Read the model definition and answer for the solid it produces. Units are mm, in the model's axes. A direction names the side the tool comes from. Coordinates: 2 decimals unless noted, no trailing zeros. Write each loop counter-clockwise with the first axis right and the second up, starting at its lowest first coordinate (ties: lowest second). Pieces come first, ordered by that corner, then holes. Notation, with made-up numbers: (33, 24) - (44, 24) arc R20 ccw to (44, 59) - close; hole circle Ø6 at (-28.75, 8). An arc over 180 degrees is marked (long way). Return JSON: item names as keys, results as strings.
Autodesk Inventor part; units mm, degrees
ref_plane "YZ Plane" through (0, 0, 0) normal (1, 0, 0) x (0, 1, 0)
ref_plane "XZ Plane" through (0, 0, 0) normal (0, 1, 0) x (-1, 0, 0)
ref_plane "XY Plane" through (0, 0, 0) normal (0, 0, 1) x (1, 0, 0)
sketch "Sketch1" plane through (0, 0, 0) normal (0, 1, 0) x (-1, 0, 0)
  line L0 (0, 0) -> (20, 0)
  line L1 (20, 0) -> (20, -20)
  line L2 (20, -20) -> (0, -20)
  line L3 (0, -20) -> (0, 0)
  dimension "d0" = 20
  dimension "d1" = 20
extrude "Extrusion1" add sketch "Sketch1" along normal blind 1
sketch "Sketch2" plane through (0, 1, 0) normal (0, 1, 0) x (1, 0, 0)
  line L0 (-15.5, 4.5) -> (-4.5, 4.5) construction
  line L1 (-4.5, 4.5) -> (-4.5, 15.5) construction
  line L2 (-4.5, 15.5) -> (-15.5, 15.5) construction
  line L3 (-15.5, 15.5) -> (-15.5, 4.5) construction
  line L4 (0, 0) -> (0, 20)
  line L5 (0, 20) -> (-20, 20)
  line L6 (-15.25, 15.25) -> (-4.75, 15.25)
  line L7 (-4.75, 15.25) -> (-4.75, 4.75)
  line L8 (-4.75, 4.75) -> (-15.25, 4.75)
  line L9 (-15.25, 4.75) -> (-15.25, 15.25)
  dimension "d4" = 11
  dimension "d5" = 11
  dimension "d6" = 4.5
  dimension "d7" = 4.5
  dimension "d20" = 0.25
extrude "Extrusion2" add sketch "Sketch2" along normal blind 1
sketch "Sketch3" plane through (0, 1, 0) normal (0, 1, 0) x (1, 0, 0)
  line L0 (-4.5, 14) -> (-3, 14)
  line L1 (-3, 14) -> (-3, 6)
  line L2 (-3, 6) -> (-4.5, 6)
  line L3 (-4.5, 6) -> (-4.5, 14)
  line L4 (-4.5, 4.5) -> (-4.5, 15.5)
  line L5 (-4.5, 15.5) -> (-15.5, 15.5)
  line L6 (-15.5, 14) -> (-17, 14)
  line L7 (-17, 14) -> (-17, 6)
  line L8 (-17, 6) -> (-15.5, 6)
  line L9 (-15.5, 6) -> (-15.5, 14)
  line L10 (-15.5, 15.5) -> (-15.5, 4.5)
  line L11 (-15.5, 4.5) -> (-4.5, 4.5)
  point P0 (0, 0)
  dimension "d10" = 8
  dimension "d11" = 1.5
  dimension "d12" = 0
  dimension "d13" = 1.5
  dimension "d14" = 8
  dimension "d15" = 1.5
  dimension "d16" = 0
  dimension "d17" = 1.5
extrude "Extrusion3" cut sketch "Sketch3" against normal through all contours L0 L1 L2 L3 | L9 L8 L7 L6
properties part number "Test_Button_Backboard"
(1) A cutting plane is placed at C-C (y = 0.25). Determine the outline of the cut face in (x, z).
Answer:
{"outline": "(-20, -20) - (0, -20) - (0, 0) - (-20, 0) - close; hole (-17, -14) - (-15.5, -14) - (-15.5, -6) - (-17, -6) - close; hole (-4.5, -14) - (-3, -14) - (-3, -6) - (-4.5, -6) - close"}
(2) A cutting plane is placed at A-A (x = -4). Determine the outline of the cut face in (y, z), and give its area (3 significant figures).
Answer:
{"outline": "(0, -20) - (1, -20) - (1, -14) - (0, -14) - close; (0, -6) - (1, -6) - (1, 0) - (0, 0) - close", "area": "12.0 mm²"}
(3) A cutting plane is placed at D-D (x = -10). Determine the outline of the cut face in (y, z).
Answer:
{"outline": "(0, -20) - (1, -20) - (1, -15.25) - (2, -15.25) - (2, -4.75) - (1, -4.75) - (1, 0) - (0, 0) - close"}
(4) Flat-ended cylindrical pins translate along their axes: P1, Ø0.8, axis at y = 1.5, z = -7.5, coming from the +X side; P2, Ø0.5, axis at x = -11, y = 1.5, coming from the +Z side; P3, Ø0.5, axis at x = -8, y = 1.5, coming from the -Z side. Find the tip coordinate at first contact, or state that the pin passes through.
Answer:
{"P1": "x = -4.75", "P2": "z = -4.75", "P3": "z = -15.25"}
(5) Determine the mould class of faces 6 (the face through (-10.1, 1.5, -15.25)), 7 (the face through (-16.3, 0.5, -6)), 8 (the face through (-3, 0.5, -10.1)), 9 (the face through (-20, 0.5, -9.9)) for opening direction Z: +Z half, -Z half, draft (parallel to the pull), parting line (faces both ways), or undercut.
Answer:
{"face 6": "-Z half", "face 7": "undercut", "face 8": "undercut", "face 9": "draft"}
(6) Which of the six approach directions +Z, -Z, +X, -X, +Y, -Y give full straight-line access (tool end or side, diameter ignored) to faces 1 (the face through (-10.1, 0.5, -20)), 2 (the face through (-9.9, 1.5, -4.75)), 3 (the face through (-15.25, 1.5, -9.9)), 4 (the face through (-4.75, 1.5, -10.1)), 5 (the face through (-17, 0.5, -10.1))?
Answer:
{"face 1": "-Z, +X, -X, +Y, -Y", "face 2": "+Z, +X, -X, +Y", "face 3": "+Z, -Z, -X, +Y", "face 4": "+Z, -Z, +X, +Y", "face 5": "+Y, -Y"}
(7) A cutting plane is placed at B-B (z = -7.5). Determine the outline of the cut face in (x, y), and give its area (3 significant figures).
Answer:
{"outline": "(-20, 0) - (-17, 0) - (-17, 1) - (-20, 1) - close; (-15.5, 0) - (-4.5, 0) - (-4.5, 1) - (-4.75, 1) - (-4.75, 2) - (-15.25, 2) - (-15.25, 1) - (-15.5, 1) - close; (-3, 0) - (0, 0) - (0, 1) - (-3, 1) - close", "area": "27.5 mm²"}
(8) Straight lines are drawn through the part: line 1 (X direction, y = 0.2, z = -7.5); line 2 (Y direction, x = -11.5, z = -2.75); line 3 (X direction, y = 1.85, z = -9.5). For each, find the intervals that lie inside material, in ascending order. Write a range as from..to.
Answer:
{"line 1": "-20..-17, -15.5..-4.5, -3..0", "line 2": "0..1", "line 3": "-15.25..-4.75"}
